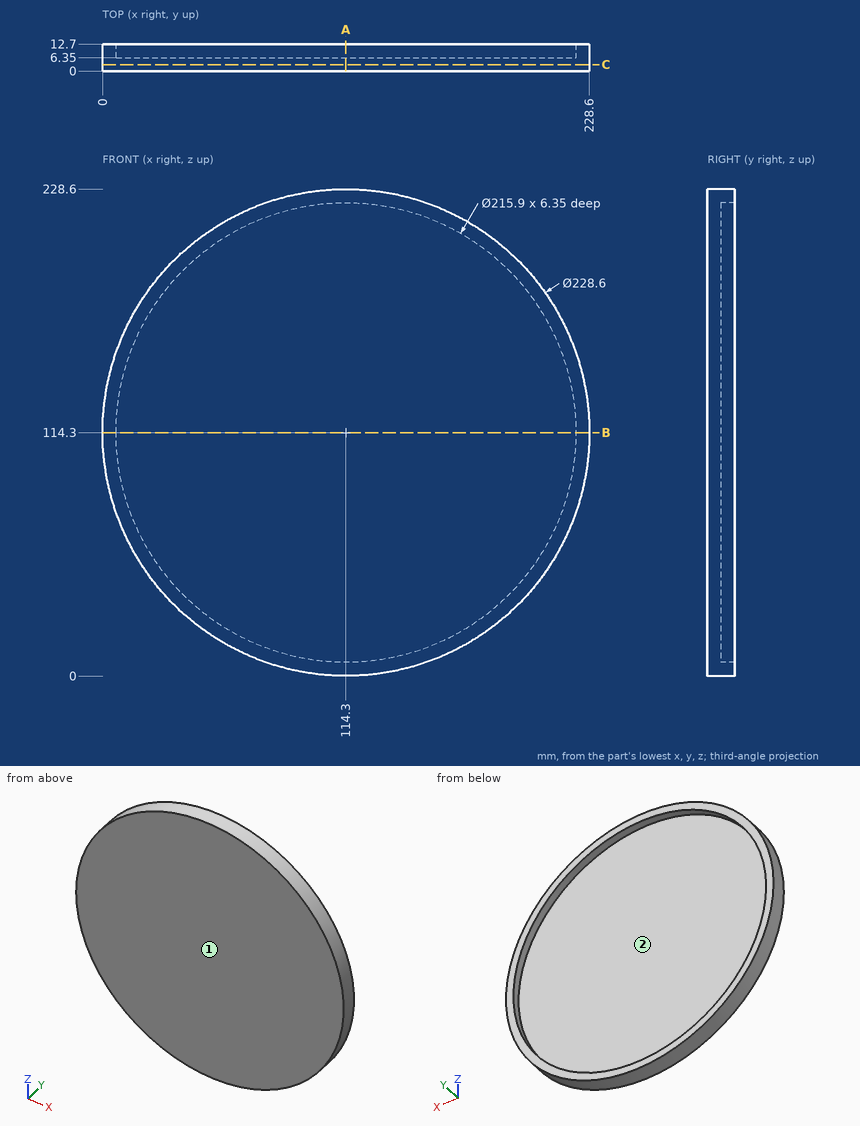
Design review of the part shown in the three views and the two pictorial views. Dimensions are in mm from the part's minimum x, y and z. Round coordinates to 2 decimals unless told otherwise and drop trailing zeros. Write each loop counter-clockwise with the first axis right and the second up, starting at its lowest first coordinate (ties: lowest second). Pieces come first, ordered by that corner, then holes. Notation, with made-up numbers: M -39.5,-6.5 L 4.5,-6.5 A16 cw 4.5,14.5 Z; hole C 26.5,77 d1. An arc over 180 degrees is marked long. One line per item, written item: value. Start each with the question number.
1. To check wall thickness, follow probe 1 along Z at (x, y) = (114.3, 11); probe 2 along Y at (x, z) = (89, 96); probe 3 along Z at (x, y) = (185.5, 8.25). State the ranges of each line that lie inside material, in increasing order. Write a range as from..to.
2. Take a section at C-C on y = 3. State the section outline as (x, z) points, then the cut area to 3 significant figures.
3. Take a section at A-A on x = 114.3. State the section outline as (y, z) points, then the cut area to 3 significant figures.
4. Clearance check with flat-ended pins moving along their axes: P1, Ø4, axis at x = 157, y = 9, coming from the -Z side; P2, Ø12, axis at x = 178, z = 149.5, coming from the +Y side; P3, Ø5, axis at x = 127, y = 3.5, coming from the +Z side. State where each tip first meets the part, or that it passes through.
5. Draft analysis for pull direction X (two halves, no side actions). For the marked faces 1 and 2, state which applies: pulls with the +X half, pulls with the -X half, needs draft (parallel to the pull), parting line crosses it, or undercut.
6. Take a section at B-B on z = 114.3. State the section outline as (x, y) points.
Computed:
1. probe 1: z = 0..6.35, 222.25..228.6
1. probe 2: y = 0..6.35
1. probe 3: z = 24.88..33.16, 195.44..203.72
2. outline: C 114.3,114.3 d228.6
2. area: 41,000 mm²
3. outline: M 0,0 L 12.7,0 L 12.7,6.35 L 6.35,6.35 L 6.35,222.25 L 12.7,222.25 L 12.7,228.6 L 0,228.6 Z
3. area: 1,530 mm²
4. P1: stops at z = 7.49
4. P2: stops at y = 6.35
4. P3: stops at z = 228.14
5. face 1: needs draft
5. face 2: undercut
6. outline: M 0,0 L 228.6,0 L 228.6,12.7 L 222.25,12.7 L 222.25,6.35 L 6.35,6.35 L 6.35,12.7 L 0,12.7 Z
